Could you check a few things on this model? Use its own coordinates, in mm. A direction names the side the tool comes from. Give positions to 0.01 mm unless a question says otherwise; leave off trailing zeros. Loops run counter-clockwise (first coordinate to the right, second up) from the corner with the lowest first, then second, coordinate; pieces in that order, holes last. Notation, with made-up numbers: M 31.25,49 L 71.25,49 A16 ccw 71.25,77 Z; hole C 31.5,70.25 d9. An arc over 180 degrees is marked long. Use a Markdown table: item, result. Add a question column.
1) We'd pull the mould along Z, two halves only. Please class faces 1 (the flat face through (-134, -110, 3)), 2 (the flat face through (-134, -113, 0)), 3 (the flat face through (-135.5, -114, 3)): +Z half, -Z half, draft (parallel to the pull), parting line (faces both ways), or undercut.
2) Suppose I cut it at C-C on x = -138.75. List the corners of the cut face in (y, z) for me, and give its area (3 significant figures).
3) Which directions (+Z, -Z, +X, -X, +Y, -Y) give clear straight access to the entire face, cutting with the end or side of a thin tool? Please do faces 4 (the cylindrical face through (-139, -116, 3.5)), 5 (the flat face through (-145.5, -115, 3)), 6 (the flat face through (-134, -113, 7)).
4) If I drill on line 1 along X through (y, z) = (-115, 1.75); line 2 along Z through (x, y) = (-125.25, -116.5); line 3 along X through (y, z) = (-115.5, 3), over which ranges is the centre line in solid material (lowest first)? Write a range as [from, to].
5) Will this pin go through, and if not, where does the flat tip stop? pin 1 Ø1.5 at (x, z) = (-144, 3) entering from -Y.
6) Suppose I cut it at B-B on z = 3.5. List the corners of the cut face in (x, y) for me, and give its area (3 significant figures).
7) Suppose I cut it at A-A on y = -114. List the corners of the cut face in (x, z) for me, and give its area (3 significant figures).
8) Suppose I cut it at D-D on y = -115.25. List the corners of the cut face in (x, z) for me, and give its area (3 significant figures).
```python
from build123d import *

# Parameters (mm, degrees)
SKETCH041_W      = 26
SKETCH041_H      = 7
EXTRUDE032_DEPTH = 7
SKETCH070_W      = 3
SKETCH070_H      = 4
POCKET012_DEPTH  = 4
SKETCH071_R      = 0.75
HOLE017_DEPTH    = 24


with BuildPart() as part:
    # Sketch041 → Extrude032 (new body)
    with BuildSketch(Plane.XY):
        with Locations((-134, -113.5)):
            Rectangle(SKETCH041_W, SKETCH041_H)
    extrude(amount=EXTRUDE032_DEPTH)

    # Sketch070 (on Face3 of BaseFeature013) → Pocket012 (cut)
    with BuildSketch(Plane.XZ.offset(117)):
        with Locations((-134.000002, 3.5)):
            Rectangle(SKETCH070_W, SKETCH070_H)
        with Locations((-144.000002, 3.5)):
            Rectangle(SKETCH070_W, SKETCH070_H)
        with Locations((-124.000002, 3.5)):
            Rectangle(SKETCH070_W, SKETCH070_H)
    extrude(amount=-POCKET012_DEPTH, mode=Mode.SUBTRACT)

    # Sketch071 (on Face3 of Pocket012) → Hole017 (cut)
    with BuildSketch(Plane.YZ.offset(-121)):
        with Locations((-115.249997, 3.5)):
            Circle(SKETCH071_R)
    extrude(amount=-HOLE017_DEPTH, mode=Mode.SUBTRACT)


solid = part.part
```
Answer block:
| question | item | result |
|---|---|---|
| 1 | face 1 | draft |
| 1 | face 2 | -Z half |
| 1 | face 3 | undercut |
| 2 | outline | M -117,0 L -110,0 L -110,7 L -117,7 Z; hole C -115.25,3.5 d1.5 |
| 2 | area | 47.2 mm^2 |
| 3 | face 4 | +X |
| 3 | face 5 | -Y |
| 3 | face 6 | +Z, +X, -X, +Y, -Y |
| 4 | line 1 | x = [-147, -145.5], [-142.5, -135.5], [-132.5, -125.5], [-122.5, -121] |
| 4 | line 2 | z = [0, 1.5], [5.5, 7] |
| 4 | line 3 | x = [-147, -145.5] |
| 5 | pin 1 | stops at y = -113 |
| 6 | outline | M -147,-117 L -145.5,-117 L -145.5,-113 L -142.5,-113 L -142.5,-114.5 L -135.5,-114.5 L -135.5,-113 L -132.5,-113 L -132.5,-114.5 L -125.5,-114.5 L -125.5,-113 L -122.5,-113 L -122.5,-114.5 L -121,-114.5 L -121,-110 L -147,-110 Z; M -142.5,-117 L -135.5,-117 L -135.5,-116 L -142.5,-116 Z; M -132.5,-117 L -125.5,-117 L -125.5,-116 L -132.5,-116 Z; M -122.5,-117 L -121,-117 L -121,-116 L -122.5,-116 Z |
| 6 | area | 123 mm^2 |
| 7 | outline | M -147,0 L -121,0 L -121,7 L -147,7 Z; hole M -145.5,1.5 L -142.5,1.5 L -142.5,5.5 L -145.5,5.5 Z; hole M -135.5,1.5 L -132.5,1.5 L -132.5,5.5 L -135.5,5.5 Z; hole M -125.5,1.5 L -122.5,1.5 L -122.5,5.5 L -125.5,5.5 Z |
| 7 | area | 146 mm^2 |
| 8 | outline | M -147,0 L -121,0 L -121,2.75 L -122.5,2.75 L -122.5,1.5 L -125.5,1.5 L -125.5,2.75 L -132.5,2.75 L -132.5,1.5 L -135.5,1.5 L -135.5,2.75 L -142.5,2.75 L -142.5,1.5 L -145.5,1.5 L -145.5,5.5 L -142.5,5.5 L -142.5,4.25 L -135.5,4.25 L -135.5,5.5 L -132.5,5.5 L -132.5,4.25 L -125.5,4.25 L -125.5,5.5 L -122.5,5.5 L -122.5,4.25 L -121,4.25 L -121,7 L -147,7 Z |
| 8 | area | 123 mm^2 |
